Autodesk Inventor part; units mm, degrees
ref_plane "Start Plane" through (0, 0, 6.314) normal (0, 0, 1) x (1, 0, 0)
ref_plane "End Plane" through (0, 0, 1337.9364) normal (0, 0, 1) x (1, 0, 0)
ref_plane "Work Plane4" through (-4.0481, -350, 17.018) normal (0.699, 0, -0.7152) x (-0.7152, 0, -0.699)
ref_plane "Start Plane" through (0, 0, 6.314) normal (0, 0, 1) x (1, 0, 0)
ref_plane "End Plane" through (0, 0, 1337.9364) normal (0, 0, 1) x (1, 0, 0)
sketch "Sketch" plane through (0, 0, 0) normal (0, 0, 1) x (1, 0, 0)
  line L0 (-15, -9) -> (-15, 9)
  line L1 (-9, 15) -> (9, 15)
  line L2 (15, 9) -> (15, -9)
  line L3 (9, -15) -> (-9, -15)
  arc A0 (-15, -9) -> (-9, -15) centre (-9, -9) ccw
  arc A1 (-9, 15) -> (-15, 9) centre (-9, 9) ccw
  arc A2 (15, 9) -> (9, 15) centre (9, 9) ccw
  arc A3 (9, -15) -> (15, -9) centre (9, -9) ccw
  arc A4 (-9, 12) -> (-12, 9) centre (-9, 9) ccw
  line L4 (-9, 12) -> (9, 12)
  arc A5 (12, 9) -> (9, 12) centre (9, 9) ccw
  line L5 (12, 9) -> (12, -9)
  arc A6 (9, -12) -> (12, -9) centre (9, -9) ccw
  line L6 (9, -12) -> (-9, -12)
  arc A7 (-12, -9) -> (-9, -12) centre (-9, -9) ccw
  line L7 (-12, -9) -> (-12, 9)
  line L8 (0, 22.7397) -> (0, -22.7397) construction
  line L9 (-22.7397, 0) -> (22.7397, 0) construction
  dimension "d7" = 6
  dimension "d10" = 30
  dimension "d11" = 30
  dimension "d12" = 3
  dimension "d15" = 15
  dimension "d16" = 15
extrude "Body" add sketch "Sketch" along normal up to surface (1331.6224 mm away) from surface at 6.314
sketch "Sketch3" plane through (0, 0, 0) normal (0, 0, 1) x (1, 0, 0)
  line L0 (0, 0) -> (10, 0)
ref_plane "Work Plane3" through (0, 0, 0) normal (0, -1, 0) x (1, 0, 0)
ref_plane "Work Plane4" through (-4.0481, -350, 17.018) normal (0.699, 0, -0.7152) x (-0.7152, 0, -0.699)
split "Split1" plane through (-4.0481, -350, 17.018) removes the side toward (0.699, 0, -0.7152)
ref_plane "Work Plane5" through (10.4845, -9, 1348.421) normal (-0.699, 0, 0.7152) x (0.7152, 0, 0.699)
split "Split2" plane through (10.4845, -9, 1348.421) removes the side toward (-0.699, 0, 0.7152)
ref_plane "Work Plane6" through (-10.7273, 9, 1348.6638) normal (0.7152, 0, 0.699) x (0.699, 0, -0.7152)
split "Split3" plane through (-10.7273, 9, 1348.6638) removes the side toward (0.7152, 0, 0.699)
sketch "Sketch4" plane through (0, 0, 0) normal (0, -1, 0) x (1, 0, 0)
  line L0 (-2, 6.314) -> (12, 6.314)
  line L1 (-2, 1337.9364) -> (12, 1337.9364)
  dimension "d18" = 1331.6224
equation "\"d7\" = G_IR"
equation "\"d10\" = G_H"
equation "\"d11\" = G_W"
equation "\"d12\" = G_T"
equation "\"d15\" = 0.5 * d10"
equation "\"d16\" = 0.5 * d11"
equation "\"d3\" = G_L"
equation "\"G_W\" = 30"
equation "\"G_H\" = 30"
equation "\"G_T\" = 3"
equation "\"G_IR\" = 6"
equation "\"G_L\" = d18"
equation "\"G_OFFSET_START\" = -6.31402"
equation "\"G_OFFSET_END\" = -21.21181"
equation "\"d13\" = -G_OFFSET_START"
equation "\"d14\" = G_OFFSET_END + B_L"
equation "\"B_L\" = 1359.14826"
properties part number "DIN EN 10219-2 - 30 x 30 x 3  - 1331.62" material "Steel, Mild"
The model under review builds one solid part; all positions refer to its coordinate system, in mm. Give positions to 0.01 mm unless a question says otherwise; leave off trailing zeros. Order: outer loops, then holes, each group sorted by start corner. A loop starts at its lowest first (then second) coordinate and runs counter-clockwise, first axis right, second up. Notation, with made-up numbers: M -2.75,32 L 43.25,32 A30 ccw 43.25,54 Z; hole C 25,39 d9. An arc over 180 degrees is marked long. One line per question, with ' | ' between items. Start each with the question number.
1) Clearance check with a flat-ended pin moving along its axis: P1, Ø3, axis at x = -11, y = 0, coming from the -Z side. State where the tip first meets the part, or that it passes through.
2) Wall thickness on L1, parallel to Y at x = -2.5, z = 619; L2, parallel to Z at x = 12, y = 11: over which ranges is each line inside the solid? List them lowest first. Write a range as from..to.
3) Consider section B-B, the plane z = 317. Give the boundary of the cut face in (x, y).
4) Consider section A-A, the plane y = -4.5. Give the boundary of the cut face in (x, z).
Found:
1) P1: stops at z = 8.76
2) L1: y = -15..-12, 12..15 | L2: z = 32.7..1325.41
3) outline: M -15,-9 A6 ccw -9,-15 L 9,-15 A6 ccw 15,-9 L 15,9 A6 ccw 9,15 L -9,15 A6 ccw -15,9 Z; hole M -12,-9 A3 ccw -9,-12 L 9,-12 A3 ccw 12,-9 L 12,9 A3 ccw 9,12 L -9,12 A3 ccw -12,9 Z
4) outline: M -15,6.31 L -12,9.25 L -12,1326.45 L -15,1323.51 Z; M 12,32.7 L 15,35.63 L 15,1322.34 L 12,1325.41 Z
